The model under review builds one solid part; all positions refer to its coordinate system, in mm. Coordinates: 2 decimals unless noted, no trailing zeros. Loops run counter-clockwise (first coordinate to the right, second up) from the corner with the lowest first, then second, coordinate; pieces in that order, holes last. Notation, with made-up numbers: (-21.5, 70.5) -> (-0.5, 70.5) arc R28 ccw to (-0.5, 92.5) -> close; hole circle Ø2 at (-10, 15). An arc over 180 degrees is marked (long way). One line per question, with ' | ' between items. Start each with the question number.
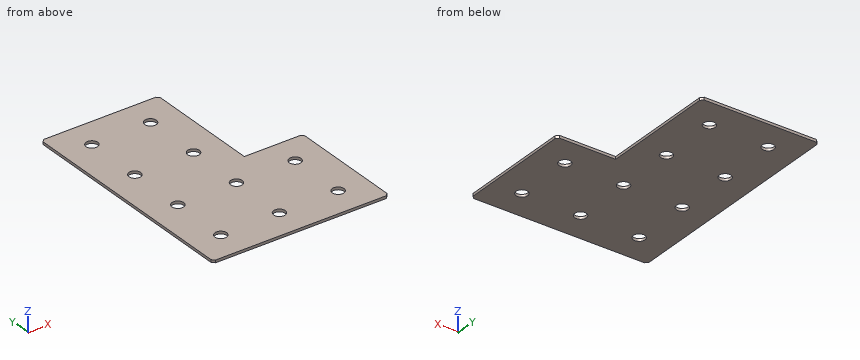
from build123d import *

# Parameters (mm, degrees)
EXTRUDE_1_DEPTH   = 2
HOLE_WIZARD_M81_D = 9
CHAMFER_1_SIZE    = 2


with BuildPart() as part:
    # Эскиз1 → Бобышка-Вытянуть1 (new body)
    with BuildSketch(Plane(origin=(0, 0, 0), x_dir=(1, 0, 0), z_dir=(0, 0, -1))):
        Polygon((0, 0), (0, 180), (135, 180), (135, 90), (90, 90), (90, 0), align=None)
    extrude(amount=EXTRUDE_1_DEPTH)

    # Отверстие с зазором M81 (through all)
    with Locations(Plane(origin=(0, 0, -2), x_dir=(1, 0, 0), z_dir=(0, 0, -1))):
        with Locations((22.5, 157.5), (22.5, 112.5), (22.5, 67.5), (22.5, 22.5), (67.5, 157.5), (67.5, 112.5), (67.5, 67.5), (67.5, 22.5), (112.5, 157.5), (112.5, 112.5)):
            Hole(HOLE_WIZARD_M81_D / 2)

    # Фаска1
    chamfer_1_edges = [part.edges().sort_by_distance(p)[0] for p in [
        (0, 0, -1),
        (0, -180, -1),
        (135, -180, -1),
        (135, -90, -1),
        (90, 0, -1),
    ]]
    chamfer(chamfer_1_edges, length=CHAMFER_1_SIZE)


solid = part.part
1) Consider section A-A, the plane x = 112.5. Write out the cut boundary in (y, z).
2) Consider section C-C, the plane x = 67.5. Write out the cut boundary in (y, z).
3) Consider section D-D, the plane y = -22.5. Write out the cut boundary in (x, z).
4) Insertion check: pin 1 Ø1 at (y, z) = (-41.5, -0.5) entering from +X. The pin has a flat end and moves straight along its axis. Give the tip position at first contact, or say it passes through.
5) Consider section B-B, the plane y = -112.5. Write out the cut boundary in (x, z), plus the area to 3 significant figures.
6) Wall thickness on L1, parallel to X at y = -112.5, z = -0.7; L2, parallel to Y at x = 67.5, z = -1.15; L3, parallel to X at y = -67.5, z = -0.6: over which ranges is each line inside the solid? List them lowest first.
Filled sheet:
1) outline: (-180, -2) -> (-162, -2) -> (-162, 0) -> (-180, 0) -> close; (-153, -2) -> (-117, -2) -> (-117, 0) -> (-153, 0) -> close; (-108, -2) -> (-90, -2) -> (-90, 0) -> (-108, 0) -> close
2) outline: (-180, -2) -> (-162, -2) -> (-162, 0) -> (-180, 0) -> close; (-153, -2) -> (-117, -2) -> (-117, 0) -> (-153, 0) -> close; (-108, -2) -> (-72, -2) -> (-72, 0) -> (-108, 0) -> close; (-63, -2) -> (-27, -2) -> (-27, 0) -> (-63, 0) -> close; (-18, -2) -> (0, -2) -> (0, 0) -> (-18, 0) -> close
3) outline: (0, -2) -> (18, -2) -> (18, 0) -> (0, 0) -> close; (27, -2) -> (63, -2) -> (63, 0) -> (27, 0) -> close; (72, -2) -> (90, -2) -> (90, 0) -> (72, 0) -> close
4) pin 1: x = 90
5) outline: (0, -2) -> (18, -2) -> (18, 0) -> (0, 0) -> close; (27, -2) -> (63, -2) -> (63, 0) -> (27, 0) -> close; (72, -2) -> (108, -2) -> (108, 0) -> (72, 0) -> close; (117, -2) -> (135, -2) -> (135, 0) -> (117, 0) -> close | area: 216 mm^2
6) L1: 0 to 18, 27 to 63, 72 to 108, 117 to 135 | L2: -180 to -162, -153 to -117, -108 to -72, -63 to -27, -18 to 0 | L3: 0 to 18, 27 to 63, 72 to 90
